Source: CAD feature listing. Evaluate the final solid. Frame: model axes, mm. A direction names the side the tool comes from. Round coordinates to 2 decimals unless told otherwise and drop trailing zeros. Write each loop counter-clockwise with the first axis right and the second up, starting at its lowest first coordinate (ties: lowest second). Pieces come first, ordered by that corner, then holes. Notation, with made-up numbers: M 68,-8 L 122,-8 A12 ccw 122,13 Z; hole C 12.5,-7.75 d8. An arc over 180 degrees is marked long. Answer in a Markdown table with one row per item.
from build123d import *

# Parameters (mm, degrees)
SKETCH_1_W      = 249
SKETCH_1_H      = 28.996988848
EXTRUDE_1_DEPTH = 4
SKETCH_2_W      = 20
SKETCH_2_H      = 4
EXTRUDE_2_DEPTH = 5.5


with BuildPart() as part:
    # Эскиз1 → Бобышка-Вытянуть1 (new body)
    with BuildSketch(Plane(origin=(0, 0, 0), x_dir=(1, 0, 0), z_dir=(0, 1, 0))):
        Rectangle(SKETCH_1_W, SKETCH_1_H)
    extrude(amount=EXTRUDE_1_DEPTH)

    # Эскиз2 → Бобышка-Вытянуть2 (add)
    with BuildSketch(Plane(origin=(124.5, 0, 0), x_dir=(0, 0, -1), z_dir=(1, 0, 0))):
        with Locations((0, 2)):
            Rectangle(SKETCH_2_W, SKETCH_2_H)
    extrude_2 = extrude(amount=EXTRUDE_2_DEPTH)

    # Mirror1: Бобышка-Вытянуть2 across plane
    add(extrude_2.mirror(Plane(origin=(0, 0, 0), x_dir=(0, 0, 1), z_dir=(1, 0, 0))))


solid = part.part
Q1. Contact query for flat-ended pins moving along their axis: pin 1 Ø2 at (y, z) = (2.5, 13.5) entering from +X; pin 2 Ø4 at (x, z) = (-10.5, 5.5) entering from -Y; pin 3 Ø1.2 at (x, y) = (-126, 1.5) entering from -Z; pin 4 Ø1.2 at (y, z) = (2, 13) entering from -X. Output: stop coordinate, or through.
Solutions:
| item | result |
|---|---|
| pin 1 | stops at x = 124.5 |
| pin 2 | stops at y = 0 |
| pin 3 | stops at z = -10 |
| pin 4 | stops at x = -124.5 |
Q2. Material intervals for probe 1 along X at (y, z) = (1.55, -12.5), sorted ascending.
Solutions:
| item | result |
|---|---|
| probe 1 | x = -124.5 to 124.5 |
Q3. Section A-A (z = -12.25). Return loops of the section in (x, y), and give its area (3 significant figures).
Solutions:
| item | result |
|---|---|
| outline | M -124.5,0 L 124.5,0 L 124.5,4 L -124.5,4 Z |
| area | 996 mm2 |
Q4. Access query for faces 1 (the flat face through (-124.5, 2, 12)), 2 (the flat face through (-124.5, 2, -12)), 3 (the flat face through (124.5, 2, 12)). Directions: +Z, -Z, +X, -X, +Y, -Y. A direction counts if a zero-diameter tool reaches every point of the face in a straight line with its end or side. Return the directions, or none.
Solutions:
| item | result |
|---|---|
| face 1 | +Z, -X, +Y, -Y |
| face 2 | -Z, -X, +Y, -Y |
| face 3 | +Z, +X, +Y, -Y |
